Source: CAD feature listing. Evaluate the final solid. Frame: model axes, mm. A direction names the side the tool comes from. Round coordinates to 2 decimals unless told otherwise and drop trailing zeros. Loops run counter-clockwise (first coordinate to the right, second up) from the corner with the lowest first, then second, coordinate; pieces in that order, holes last. Notation, with made-up numbers: (28, 29.25) -> (54, 29.25) arc R12 ccw to (54, 45.25) -> close; hole circle Ø9 at (72, -18). An arc over 180 degrees is marked (long way). Put each result on its own line as item: value. Start each with the question number.
1. Cut plane B-B (y = 4). Return the cut outline in (x, z).
2. Cut plane C-C (x = -3). Return the cut outline in (y, z) (3 decimals), then the cut area to 3 significant figures.
3. Material intervals for L1, parallel to X at y = 0.5, z = 4.25; L2, parallel to X at y = 6.5, z = 3.75; L3, parallel to Z at x = 0, y = 10.5, sorted ascending.
4. Draft query along X for faces 3 (the flat face through (17.143, 5, 8)), 4 (the flat face through (-5.577, 5.322, 3.565)), 5 (the flat face through (0, 10.795, 8)). Return one class per face: pulls with the +X half, pulls with the -X half, needs draft (parallel to the pull), parting line crosses it, or undercut.
5. Set-up query: faces 1 (the flat face through (0, 0, 8)), 2 (the flat face through (5.63, 5.32, 3.51)). Return all of +Z, -Z, +X, -X, +Y, -Y with unobstructed straight access to the full face (end or side cutting, diameter ignored); none if empty.
6. Cut plane A-A (z = 3.75). Return the cut outline in (x, y) (3 decimals).
```python
from build123d import *

# Parameters (mm, degrees)
BOSS_EXTRUDE1_DEPTH = 10.795
FILLET1_R           = 5.08


with BuildPart() as part:
    # Sketch1 → Boss-Extrude1 (new body)
    with BuildSketch(Plane(origin=(0, 0, 0), x_dir=(1, 0, 0), z_dir=(0, 1, 0))):
        Polygon((7.617900731, -1.524), (0, -9.141900731), (-7.617900731, -1.524), (-17.142900731, -1.524), (-17.142900731, -14.221900731), (17.142900731, -14.221900731), (17.142900731, -1.524), align=None)
    extrude(amount=BOSS_EXTRUDE1_DEPTH)

    # Fillet1
    fillet1_edges = [part.edges().sort_by_distance(p)[0] for p in [
        (0, 5.3975, 9.141900731),
    ]]
    fillet(fillet1_edges, radius=FILLET1_R)


solid = part.part
```
Solution:
1. outline: (-17.14, 1.52) -> (-7.62, 1.52) -> (-3.59, 5.55) arc R5.08 cw to (3.59, 5.55) -> (7.62, 1.52) -> (17.14, 1.52) -> (17.14, 14.22) -> (-17.14, 14.22) -> close
2. outline: (0, 6.057) -> (10.795, 6.057) -> (10.795, 14.222) -> (0, 14.222) -> close
2. area: 88.1 mm^2
3. L1: x = -17.14 to -4.89, 4.89 to 17.14
3. L2: x = -17.14 to -5.39, 5.39 to 17.14
3. L3: z = 7.04 to 14.22
4. face 3: pulls with the +X half
4. face 4: undercut
4. face 5: needs draft
5. face 1: +Z, -Z, +X, -X, -Y
5. face 2: -Z, +Y, -Y
6. outline: (-17.143, 0) -> (-5.392, 0) -> (-5.392, 10.795) -> (-17.143, 10.795) -> close; (5.392, 0) -> (17.143, 0) -> (17.143, 10.795) -> (5.392, 10.795) -> close
